from build123d import *

# Parameters (mm, degrees)
BOSS_EXTRUDE1_DEPTH      = 11.5
CUT_EXTRUDE1_DEPTH       = 35.906446396
CUT_EXTRUDE1_DEPTH_BACK  = 35.906446396
SKETCH3_R                = 1.05
BOSS_EXTRUDE2_DEPTH      = 3
BOSS_EXTRUDE2_DEPTH_BACK = 11.5
SKETCH4_W                = 3.75
SKETCH4_H                = 3
CUT_EXTRUDE2_DEPTH       = 38.275461128
CUT_EXTRUDE2_DEPTH_BACK  = 38.275461128
SKETCH5_R                = 1.25
CHAMFER1_SIZE            = 6.528307214
CHAMFER1_SIZE_2          = 14
CHAMFER2_SIZE            = 6.528307214
CHAMFER2_SIZE_2          = 14
SKETCH6_R                = 2.6
CUT_EXTRUDE3_DEPTH       = 5
SKETCH7_R                = 1.5
CUT_EXTRUDE4_DEPTH       = 12


with BuildPart() as part:
    # Sketch1 → Boss-Extrude1 (new body)
    with BuildSketch(Plane.XY):
        with BuildLine():
            Line((16.91, 0), (18.9, 0))
            Line((18.9, 0), (18.9, 27))
            Line((18.9, 27), (-3.75, 27))
            Line((-3.75, 27), (-3.75, 0))
            Line((-3.75, 0), (-1.76, 0))
            ThreePointArc((-1.76, 0), (-0.515492065, 0.515492065), (0, 1.76))
            Line((0, 1.76), (0, 6))
            ThreePointArc((0, 6), (0.732233047, 7.767766953), (2.5, 8.5))
            Line((2.5, 8.5), (12.65, 8.5))
            ThreePointArc((12.65, 8.5), (14.417766953, 7.767766953), (15.15, 6))
            Line((15.15, 6), (15.15, 1.76))
            ThreePointArc((15.15, 1.76), (15.665492065, 0.515492065), (16.91, 0))
        make_face()
    extrude(amount=-BOSS_EXTRUDE1_DEPTH)

    # Sketch3 → Cut-Extrude1 (cut, two sides: drawn at the far end of the back side and taken through both)
    with BuildSketch(Plane(origin=(0, 27, 0), x_dir=(1, 0, 0), z_dir=(0, 1, 0)).offset(-CUT_EXTRUDE1_DEPTH_BACK)):
        with Locations(Location((-1.425, 7.25, 0), (0, 0, 251.394661296))):
            Circle(SKETCH3_R)
        with Locations(Location((16.575, 7.25, 0), (0, 0, 288.605338704))):
            Circle(SKETCH3_R)
    extrude(amount=CUT_EXTRUDE1_DEPTH + CUT_EXTRUDE1_DEPTH_BACK, mode=Mode.SUBTRACT)

    # Sketch4 → Boss-Extrude2 (add, two sides: drawn at the far end of the back side and taken through both)
    with BuildSketch(Plane.XZ.offset(-BOSS_EXTRUDE2_DEPTH_BACK)):
        with Locations((17.025, -1.5)):
            Rectangle(SKETCH4_W, SKETCH4_H)
        with Locations((-1.875, -1.5)):
            Rectangle(SKETCH4_W, SKETCH4_H)
    extrude(amount=BOSS_EXTRUDE2_DEPTH + BOSS_EXTRUDE2_DEPTH_BACK)

    # Sketch5 → Cut-Extrude2 (cut, two sides: drawn at the far end of the back side and taken through both)
    with BuildSketch(Plane(origin=(0, 27, 0), x_dir=(1, 0, 0), z_dir=(0, 1, 0)).offset(-CUT_EXTRUDE2_DEPTH_BACK)):
        with Locations(Location((7.575, 7.5, 0), (0, 0, 90))):
            Circle(SKETCH5_R)
    extrude(amount=CUT_EXTRUDE2_DEPTH + CUT_EXTRUDE2_DEPTH_BACK, mode=Mode.SUBTRACT)

    # Chamfer1
    # the kernel refuses this chamfer: 14, 6.528307214 mm, written as the material it takes off along each edge
    with BuildSketch(Plane(origin=(-3.75, 27, 36.2736566), x_dir=(0.9971975577536776, 0.07481330637059945, 0), z_dir=(0, 0, -1))) as chamfer1_piece_1:
        Polygon((CHAMFER1_SIZE * 0.99719755778, CHAMFER1_SIZE * 0.0748133063725), (-CHAMFER1_SIZE_2 * 0.0748133063706, CHAMFER1_SIZE_2 * 0.997197557754), (0, 0), align=None)
    extrude(amount=84.0473132, mode=Mode.SUBTRACT)

    # Chamfer2
    # the kernel refuses this chamfer: 14, 6.528307214 mm, written as the material it takes off along each edge
    with BuildSketch(Plane(origin=(18.9, 27, 36.2736566), x_dir=(-0.9971975577536776, 0.07481330637059945, 0), z_dir=(0, 0, -1))) as chamfer2_piece_1:
        Polygon((CHAMFER2_SIZE * 0.99719755778, -CHAMFER2_SIZE * 0.0748133063725), (-CHAMFER2_SIZE_2 * 0.0748133063706, -CHAMFER2_SIZE_2 * 0.997197557754), (0, 0), align=None)
    extrude(amount=84.0473132, mode=Mode.SUBTRACT)

    # Sketch6 → Cut-Extrude3 (cut)
    with BuildSketch(Plane(origin=(0, 27, 0), x_dir=(1, 0, 0), z_dir=(0, 1, 0))):
        with Locations(Location((7.575, 7.5, 0), (0, 0, 270))):
            Circle(SKETCH6_R)
    extrude(amount=-CUT_EXTRUDE3_DEPTH, mode=Mode.SUBTRACT)

    # Sketch7 → Cut-Extrude4 (cut)
    with BuildSketch(Plane(origin=(0, 27, 0), x_dir=(1, 0, 0), z_dir=(0, 1, 0))):
        with Locations((-1.425, 7.25)):
            Circle(SKETCH7_R)
        with Locations((16.575, 7.25)):
            Circle(SKETCH7_R)
    extrude(amount=-CUT_EXTRUDE4_DEPTH, mode=Mode.SUBTRACT)


solid = part.part
CAD build for the part. Positions are in the model's coordinates, mm. A direction names the side the tool comes from. Give positions to 0.01 mm unless a question says otherwise; leave off trailing zeros. Write each loop counter-clockwise with the first axis right and the second up, starting at its lowest first coordinate (ties: lowest second). Pieces come first, ordered by that corner, then holes. Notation, with made-up numbers: (65, -40) -> (109, -40) arc R30 cw to (109, -14) -> close; hole circle Ø8 at (-15.5, 64.5). An arc over 180 degrees is marked (long way). Return JSON: item names as keys, results as strings.
Item 1: Two-plate mould, pull along Z, no slides. Class faces 1 (the flat face through (8, 22, -6)), 2 (the flat face through (7, 14, -11.5)), 3 (the flat face through (18, 0, -7)): +Z half, -Z half, draft (parallel to the pull), parting line (faces both ways), or undercut.
Answer below:
{"face 1": "undercut", "face 2": "-Z half", "face 3": "draft"}
Item 2: Band-saw the part on D-D (y = 17.5). List the corners of the cut face in (x, z) (3 decimals).
Answer below:
{"outline": "(-1.652, -11.5) -> (16.802, -11.5) -> (16.802, -8.733) arc R1.5 cw (long way) to (16.802, -5.767) -> (16.802, 0) -> (-1.652, 0) -> (-1.652, -5.767) arc R1.5 cw (long way) to (-1.652, -8.733) -> close; hole circle Ø2.5 at (7.575, -7.5)"}
Item 3: Band-saw the part on C-C (z = -7.25). Give the number of separate pieces and of enclosed holes in the cut face, then the cut area to 3 significant figures.
Answer below:
{"separate pieces": "4", "enclosed holes": "0", "area": "253 mm2"}
Item 4: Band-saw the part on B-B (z = -1.5). List the corners of the cut face in (x, y), then the cut area to 3 significant figures.
Answer below:
{"outline": "(-3.75, -3) -> (0, -3) -> (0, 6) arc R2.5 cw to (2.5, 8.5) -> (12.65, 8.5) arc R2.5 cw to (15.15, 6) -> (15.15, -3) -> (18.9, -3) -> (18.9, 13) -> (12.37, 27) -> (2.78, 27) -> (-3.75, 13) -> close", "area": "417 mm2"}
Item 5: Band-saw the part on A-A (y = 5.5). List the corners of the cut face in (x, z) (3 decimals).
Answer below:
{"outline": "(-3.75, -11.5) -> (0, -11.5) -> (0, 0) -> (-3.75, 0) -> close; (15.15, -11.5) -> (18.9, -11.5) -> (18.9, 0) -> (15.15, 0) -> close; hole circle Ø2.1 at (-1.425, -7.25); hole circle Ø2.1 at (16.575, -7.25)"}
Item 6: Drill centre lines: probe 1 along X at (y, z) = (2.5, -3.75); probe 2 along Z at (x, y) = (-1.5, 16.5); probe 3 along Y at (x, z) = (11, -10.5). Where is each one in solid material? Low to high.
Answer below:
{"probe 1": "x = -3.75 to 0, 15.15 to 18.9", "probe 2": "z = -11.5 to -8.75, -5.75 to 0", "probe 3": "y = 8.5 to 27"}
Item 7: Tool access for faces 4 (the cylindrical face through (15.076, 17.547, -7.308)), 5 (the cylindrical face through (1, 8, -6)), 6 (the flat face through (7, 12, 0)), 7 (the flat face through (-3, 0, -7)), 8 (the cylindrical face through (15.31, 1.03, -7.19)): list every direction of +Z, -Z, +X, -X, +Y, -Y with a clear straight run to the whole face (end or side of a thin tool).
Answer below:
{"face 4": "+Y", "face 5": "+Z, -Z, -Y", "face 6": "+Z, +X, -X, +Y, -Y", "face 7": "-Z, +X, -X, -Y", "face 8": "-Z, -Y"}
Item 8: Drop flat-ended pins along their axis: pin 1 (2.5 mm diameter, centred on x = -1.425, z = -7.25, fed in from +Y); pin 2 (3.5 mm diameter, centred on x = 16.575, z = -7.25, fed in from -Y); pin 3 (2 mm diameter, centred on y = 20, z = -1.5, fed in from +X). Give the stop position or say it passes through.
Answer below:
{"pin 1": "stops at y = 15", "pin 2": "stops at y = 0", "pin 3": "stops at x = 16.1"}
